Check sheet for the modelled part. Datum: model origin and axes. Units: mm. A direction names the side the tool comes from. Give positions to 0.01 mm unless a question says otherwise; leave off trailing zeros. Order: outer loops, then holes, each group sorted by start corner. A loop starts at its lowest first (then second) coordinate and runs counter-clockwise, first axis right, second up. Notation, with made-up numbers: (63.25, 38.25) - (81.25, 38.25) arc R23 ccw to (81.25, 72.25) - close; hole circle Ø8 at (-15, 69.25). An arc over 180 degrees is marked (long way). Answer in a Markdown table with one row per item.
from build123d import *

# Parameters (mm, degrees)
SKETCH1_W           = 20.32
SKETCH1_H           = 45.72
BOSS_EXTRUDE1_DEPTH = 25.4
SKETCH2_R           = 2.54
CUT_EXTRUDE1_DEPTH  = 57.110433967
SKETCH3_R           = 2.54
CUT_EXTRUDE2_DEPTH  = 7.62


with BuildPart() as part:
    # Sketch1 → Boss-Extrude1 (new body)
    with BuildSketch(Plane(origin=(0, 0, 0), x_dir=(1, 0, 0), z_dir=(0, 1, 0))):
        with Locations((10.16, -22.86)):
            Rectangle(SKETCH1_W, SKETCH1_H)
    extrude(amount=BOSS_EXTRUDE1_DEPTH)

    # Sketch2 → Cut-Extrude1 (cut, through all)
    with BuildSketch(Plane.XY.offset(45.72)):
        with Locations((10.16, 12.7)):
            Circle(SKETCH2_R)
    extrude(amount=-CUT_EXTRUDE1_DEPTH, mode=Mode.SUBTRACT)

    # Sketch3 → Cut-Extrude2 (cut)
    with BuildSketch(Plane(origin=(0, 0, 0), x_dir=(-1, 0, 0), z_dir=(0, -1, 0))):
        with Locations(Location((-10.16, -35.56, 0), (0, 0, 90))):
            Circle(SKETCH3_R)
        with Locations(Location((-10.16, -10.16, 0), (0, 0, 90))):
            Circle(SKETCH3_R)
    extrude(amount=-CUT_EXTRUDE2_DEPTH, mode=Mode.SUBTRACT)


solid = part.part
(1) Gauge pin test, flat ends, axial feed: P1, Ø3, axis at y = 15, z = 30, coming from the -X side; P2, Ø1.5, axis at x = 11.5, z = 11, coming from the -Y side. Record the tip position at first contact, or that the pin passes through.
Geometry says:
| item | result |
|---|---|
| P1 | x = 0 |
| P2 | y = 7.62 |
(2) Cross-section at B-B, the plane y = 12.7. Record the cut outline in (x, z).
Geometry says:
| item | result |
|---|---|
| outline | (0, 0) - (7.62, 0) - (7.62, 45.72) - (0, 45.72) - close; (12.7, 0) - (20.32, 0) - (20.32, 45.72) - (12.7, 45.72) - close |
(3) Mould release check, pull along Y, two halves, no side actions. Record for faces 3 (the flat face through (10, 10, 45.72)), 4 (the cylindrical face through (8.29, 14.42, 23.18)), 5 (the flat face through (10, 0, 23)): pulls with the +Y half, pulls with the -Y half, needs draft (parallel to the pull), parting line crosses it, or undercut.
Geometry says:
| item | result |
|---|---|
| face 3 | needs draft |
| face 4 | undercut |
| face 5 | pulls with the -Y half |
(4) Thickness scan on L1, parallel to Y at x = 10.16, z = 35; L2, parallel to X at y = 2.75, z = 35.56. Record the ranges inside material, lowest first.
Geometry says:
| item | result |
|---|---|
| L1 | 7.62 to 10.16, 15.24 to 25.4 |
| L2 | 0 to 7.62, 12.7 to 20.32 |
(5) Cross-section at A-A, the plane x = 10.16. Record the cut outline in (y, z).
Geometry says:
| item | result |
|---|---|
| outline | (0, 0) - (10.16, 0) - (10.16, 45.72) - (0, 45.72) - (0, 38.1) - (7.62, 38.1) - (7.62, 33.02) - (0, 33.02) - (0, 12.7) - (7.62, 12.7) - (7.62, 7.62) - (0, 7.62) - close; (15.24, 0) - (25.4, 0) - (25.4, 45.72) - (15.24, 45.72) - close |
(6) Access from +Z, -Z, +X, -X, +Y, -Y to the whole of each face (thin tool, end or side, straight path). Record for faces 1 (the flat face through (0, 13, 23)), 2 (the cylindrical face through (10.923, 3.757, 7.737)).
Geometry says:
| item | result |
|---|---|
| face 1 | +Z, -Z, -X, +Y, -Y |
| face 2 | -Y |
(7) Cross-section at D-D, the plane z = 18.5. Record the cut outline in (x, y), then the cut area to 3 significant figures.
Geometry says:
| item | result |
|---|---|
| outline | (0, 0) - (20.32, 0) - (20.32, 25.4) - (0, 25.4) - close; hole circle Ø5.08 at (10.16, 12.7) |
| area | 496 mm² |
(8) Cross-section at C-C, the plane z = 10.16. Record the cut outline in (x, y).
Geometry says:
| item | result |
|---|---|
| outline | (0, 0) - (7.62, 0) - (7.62, 7.62) - (12.7, 7.62) - (12.7, 0) - (20.32, 0) - (20.32, 25.4) - (0, 25.4) - close; hole circle Ø5.08 at (10.16, 12.7) |
